Verification items for the finished model (mm, model axes). Face numbers are marked on the shaded views. Give positions to 0.01 mm unless a question says otherwise; leave off trailing zeros. Write each loop counter-clockwise with the first axis right and the second up, starting at its lowest first coordinate (ties: lowest second). Pieces come first, ordered by that corner, then holes. Notation, with made-up numbers: (18.25, 36.5) -> (48.25, 36.5) arc R7 ccw to (48.25, 44.5) -> close; hole circle Ø4 at (61.5, 26.25). An arc over 180 degrees is marked (long way). Write item = value, one per line.
from build123d import *

# Parameters (mm, degrees)
CYLINDER1752_R               = 1.5
CYLINDER1752_DEPTH           = 30
CYLINDER1752_PLACEMENT_ANGLE = 45
CYLINDER1753_R               = 1.5
CYLINDER1753_DEPTH           = 30
CYLINDER1754_R               = 1.5
CYLINDER1754_DEPTH           = 30
CYLINDER1754_PLACEMENT_ANGLE = 135
CYLINDER1750_R               = 1.5
CYLINDER1750_DEPTH           = 30
CYLINDER1748_R               = 1.5
CYLINDER1748_DEPTH           = 30
CYLINDER1748_PLACEMENT_ANGLE = 225
CYLINDER1751_R               = 1.5
CYLINDER1751_DEPTH           = 30
CYLINDER1749_R               = 1.5
CYLINDER1749_DEPTH           = 30
CYLINDER1749_PLACEMENT_ANGLE = 45
CYLINDER1755_R               = 1.5
CYLINDER1755_DEPTH           = 30
TUBE089_R                    = 35
TUBE089_R_2                  = 29.1
TUBE089_DEPTH                = 9


with BuildPart() as obj1:
    # Cylinder1752 → Cylinder1752 (new body)
    with BuildSketch(Plane.XY):
        Circle(CYLINDER1752_R)
    extrude(amount=CYLINDER1752_DEPTH)


with BuildPart() as obj1_1:
    # Cylinder1752 placement: moved
    add(obj1.part.moved(Location((22.627417, -22.627417, 0))).rotate(Axis((22.627417, -22.627417, 0), (0, 0, 1)), CYLINDER1752_PLACEMENT_ANGLE))


with BuildPart() as obj2:
    # Cylinder1753 → Cylinder1753 (new body)
    with BuildSketch(Plane(origin=(32, 0, 0), x_dir=(0, 1, 0), z_dir=(0, 0, 1))):
        Circle(CYLINDER1753_R)
    extrude(amount=CYLINDER1753_DEPTH)


with BuildPart() as obj3:
    # Cylinder1754 → Cylinder1754 (new body)
    with BuildSketch(Plane.XY):
        Circle(CYLINDER1754_R)
    extrude(amount=CYLINDER1754_DEPTH)


with BuildPart() as obj3_1:
    # Cylinder1754 placement: moved
    add(obj3.part.moved(Location((22.627417, 22.627417, 0))).rotate(Axis((22.627417, 22.627417, 0), (0, 0, 1)), CYLINDER1754_PLACEMENT_ANGLE))


with BuildPart() as obj4:
    # Cylinder1750 → Cylinder1750 (new body)
    with BuildSketch(Plane(origin=(0, 32, 0), x_dir=(-1, 0, 0), z_dir=(0, 0, 1))):
        Circle(CYLINDER1750_R)
    extrude(amount=CYLINDER1750_DEPTH)


with BuildPart() as obj5:
    # Cylinder1748 → Cylinder1748 (new body)
    with BuildSketch(Plane.XY):
        Circle(CYLINDER1748_R)
    extrude(amount=CYLINDER1748_DEPTH)


with BuildPart() as obj5_1:
    # Cylinder1748 placement: moved
    add(obj5.part.moved(Location((-22.627417, 22.627417, 0))).rotate(Axis((-22.627417, 22.627417, 0), (0, 0, 1)), CYLINDER1748_PLACEMENT_ANGLE))


with BuildPart() as obj6:
    # Cylinder1751 → Cylinder1751 (new body)
    with BuildSketch(Plane(origin=(-32, 0, 0), x_dir=(0, -1, 0), z_dir=(0, 0, 1))):
        Circle(CYLINDER1751_R)
    extrude(amount=CYLINDER1751_DEPTH)


with BuildPart() as obj7:
    # Cylinder1749 → Cylinder1749 (new body)
    with BuildSketch(Plane.XY):
        Circle(CYLINDER1749_R)
    extrude(amount=CYLINDER1749_DEPTH)


with BuildPart() as obj7_1:
    # Cylinder1749 placement: moved
    add(obj7.part.moved(Location((-22.627417, -22.627417, 0))).rotate(Axis((-22.627417, -22.627417, 0), (0, 0, -1)), CYLINDER1749_PLACEMENT_ANGLE))


with BuildPart() as compound879:
    # Cylinder1755 → Cylinder1755 (new body)
    with BuildSketch(Plane(origin=(0, -32, 0), x_dir=(1, 0, 0), z_dir=(0, 0, 1))):
        Circle(CYLINDER1755_R)
    extrude(amount=CYLINDER1755_DEPTH)

    # Compound879: union obj1, obj2, obj3, obj4, obj5, obj6, obj7
    add(obj1_1.part)
    add(obj2.part)
    add(obj3_1.part)
    add(obj4.part)
    add(obj5_1.part)
    add(obj6.part)
    add(obj7_1.part)


with BuildPart() as cut508:
    # Tube089 → Tube089 (new body)
    with BuildSketch(Plane.XY.offset(16)):
        Circle(TUBE089_R)
        Circle(TUBE089_R_2, mode=Mode.SUBTRACT)
    extrude(amount=TUBE089_DEPTH)

    # Cut508: cut Compound879
    add(compound879.part, mode=Mode.SUBTRACT)


solid = cut508.part
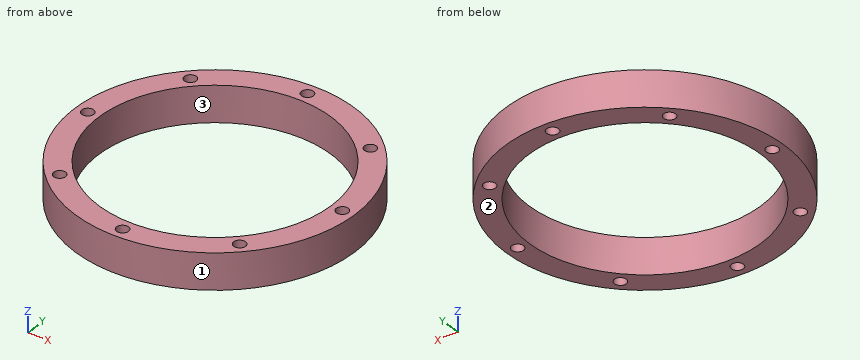
Item 1: Go/stop test with flat-tipped pins: P1, Ø4, axis at x = -26.5, y = -1.5, coming from the -Z side; P2, Ø1.5, axis at y = -27, z = 22.5, coming from the +X side; P3, Ø2, axis at y = 17, z = 19.5, coming from the +X side; P4, Ø5, axis at y = -25.5, z = 21, coming from the +X side. Record where each tip stops, or that it passes through.
Response values:
P1 = through
P2 = 23.15
P3 = 31.13
P4 = 26.38
Item 2: Mould release check, pull along X, two halves, no side actions. Record for the marked faces 1, 2 and 3: +X half, -X half, draft (parallel to the pull), parting line (faces both ways), or undercut.
Response values:
face_1 = parting line
face_2 = draft
face_3 = undercut
Item 3: Material ranges on line 1 (Y direction, x = -22, z = 22); line 2 (Y direction, x = 0, z = 20.25); line 3 (X direction, y = 23, z = 24.5), recorded low to high.
Response values:
line_1 = -27.22 to -23.99, -21.26 to -19.05, 19.05 to 21.26, 23.99 to 27.22
line_2 = -35 to -33.5, -30.5 to -29.1, 29.1 to 30.5, 33.5 to 35
line_3 = -26.38 to -24.08, -21.17 to -17.83, 17.83 to 21.17, 24.08 to 26.38
Item 4: Sectioned sample at B-B on y = -32. Record the cut outline in (x, z), then the cut area to 3 significant figures.
Response values:
outline = (-14.18, 16) -> (-1.5, 16) -> (-1.5, 25) -> (-14.18, 25) -> close; (1.5, 16) -> (14.18, 16) -> (14.18, 25) -> (1.5, 25) -> close
area = 228 mm^2
Item 5: Sectioned sample at A-A on x = 0. Record the cut outline in (y, z), then the cut area to 3 significant figures.
Response values:
outline = (-35, 16) -> (-33.5, 16) -> (-33.5, 25) -> (-35, 25) -> close; (-30.5, 16) -> (-29.1, 16) -> (-29.1, 25) -> (-30.5, 25) -> close; (29.1, 16) -> (30.5, 16) -> (30.5, 25) -> (29.1, 25) -> close; (33.5, 16) -> (35, 16) -> (35, 25) -> (33.5, 25) -> close
area = 52.2 mm^2
Item 6: Sectioned sample at C-C on x = 19. Record the cut outline in (y, z).
Response values:
outline = (-29.39, 16) -> (-22.04, 16) -> (-22.04, 25) -> (-29.39, 25) -> close; (22.04, 16) -> (29.39, 16) -> (29.39, 25) -> (22.04, 25) -> close
